Could you check a few things on this model? Use its own coordinates, in mm. Face numbers are marked on the shaded views. Give positions to 0.01 mm unless a question says otherwise; leave off trailing zeros. Write each loop counter-clockwise with the first axis right and the second up, starting at its lowest first coordinate (ties: lowest second). Pieces come first, ordered by that corner, then holes. Notation, with made-up numbers: M -29.5,-19.75 L 25.5,-19.75 A32 cw 25.5,17.25 Z; hole C 78,-19 d3. An arc over 180 degrees is marked long. Answer as CSV lines item,"result". Start each with the question number.
from build123d import *

# Parameters (mm, degrees)
SKETCH1_W         = 30
SKETCH1_H         = 30
EXTRUSION1_DEPTH  = 3.5
SKETCH2_W         = 80
SKETCH2_H         = 80
EXTRUSION2_DEPTH  = 8
EXTRUSION3_DEPTH  = 3.5
FILLET1_R         = 0.5
HOLE2_D           = 4.305
HOLE2_DEPTH       = 8
HOLE2_CBORE_D     = 7.145
HOLE2_CBORE_DEPTH = 4
HOLE2_TIP         = 1.293352482
EXTRUSION4_START  = 0.5
SKETCH6_R         = 3.5
SKETCH6_R_2       = 2.1525
EXTRUSION4_DEPTH  = 0.5


with BuildPart() as part:
    # Sketch1 → Extrusion1 (new body)
    with BuildSketch(Plane.XY):
        Rectangle(SKETCH1_W, SKETCH1_H)
    extrude(amount=EXTRUSION1_DEPTH)

    # Sketch2 → Extrusion2 (add)
    with BuildSketch(Plane(origin=(0, 0, 0), x_dir=(-1, 0, 0), z_dir=(0, 0, -1))):
        Rectangle(SKETCH2_W, SKETCH2_H)
    extrude(amount=EXTRUSION2_DEPTH)

    # Sketch3 → Extrusion3 (cut)
    with BuildSketch(Plane.XY.offset(3.5)):
        with BuildLine():
            Line((-2.292893219, -15), (2.292893219, -15))
            Line((2.292893219, -15), (2.292893219, -13.707106781))
            ThreePointArc((2.292893219, -13.707106781), (2, -13), (1.292893219, -12.707106781))
            Line((1.292893219, -12.707106781), (-1.292893219, -12.707106781))
            ThreePointArc((-1.292893219, -12.707106781), (-2, -13), (-2.292893219, -13.707106781))
            Line((-2.292893219, -13.707106781), (-2.292893219, -15))
        make_face()
    extrude(amount=-EXTRUSION3_DEPTH, mode=Mode.SUBTRACT)

    # Fillet1
    fillet1_edges = [part.edges().sort_by_distance(p)[0] for p in [
        (2.292893219, -15, 1.75),
        (-2.292893219, -15, 1.75),
        (-15, 15, 1.75),
        (15, 15, 1.75),
        (15, -15, 1.75),
        (-15, -15, 1.75),
    ]]
    fillet(fillet1_edges, radius=FILLET1_R)

    # Hole2
    with Locations(Plane(origin=(0, 0, -8), x_dir=(-1, 0, 0), z_dir=(0, 0, -1))):
        with Locations((24.525, -25.25), (24.525, 25.25), (-24.525, 25.25), (-24.525, -25.25)):
            CounterBoreHole(HOLE2_D / 2, HOLE2_CBORE_D / 2, HOLE2_CBORE_DEPTH, depth=HOLE2_DEPTH)
            with Locations((0, 0, -(HOLE2_DEPTH + HOLE2_TIP / 2))):  # 118° drill point
                Cone(0, HOLE2_D / 2, HOLE2_TIP, mode=Mode.SUBTRACT)

    # Sketch6 → Extrusion4 (add)
    # profile 1 of 4: a face of its own
    with BuildSketch(Plane.XY.offset(EXTRUSION4_START)):
        with Locations(Location((-24.525, 25.25, 0), (0, 0, 180))):
            Circle(SKETCH6_R)
        with Locations(Location((-24.525, 25.25, 0), (0, 0, 180))):
            Circle(SKETCH6_R_2, mode=Mode.SUBTRACT)
    # profile 2 of 4: a face of its own
    with BuildSketch(Plane.XY.offset(EXTRUSION4_START)):
        with Locations(Location((24.525, 25.25, 0), (0, 0, 180))):
            Circle(SKETCH6_R)
        with Locations(Location((24.525, 25.25, 0), (0, 0, 180))):
            Circle(SKETCH6_R_2, mode=Mode.SUBTRACT)
    # profile 3 of 4: a face of its own
    with BuildSketch(Plane.XY.offset(EXTRUSION4_START)):
        with Locations(Location((-24.525, -25.25, 0), (0, 0, 180))):
            Circle(SKETCH6_R)
        with Locations(Location((-24.525, -25.25, 0), (0, 0, 180))):
            Circle(SKETCH6_R_2, mode=Mode.SUBTRACT)
    # profile 4 of 4: a face of its own
    with BuildSketch(Plane.XY.offset(EXTRUSION4_START)):
        with Locations(Location((24.525, -25.25, 0), (0, 0, 180))):
            Circle(SKETCH6_R)
        with Locations(Location((24.525, -25.25, 0), (0, 0, 180))):
            Circle(SKETCH6_R_2, mode=Mode.SUBTRACT)
    extrude(amount=-EXTRUSION4_DEPTH)


solid = part.part
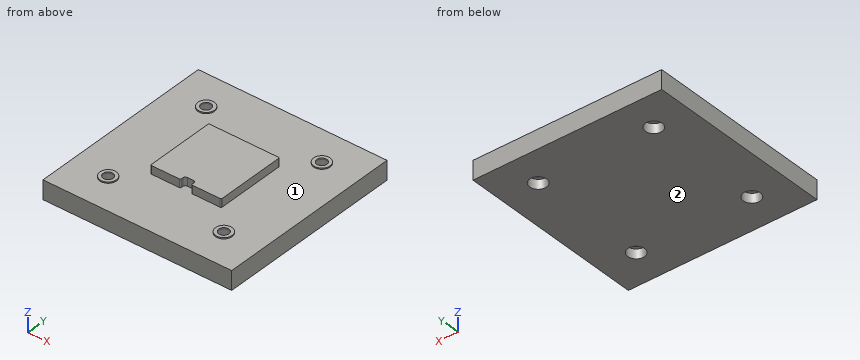
1. Imagine slicing it at A-A, the plane y = 25.25. Please give me the cut outline in (x, z) (1 decimal).
2. Please list where these lines run through material, in increasing order: line 1 (X direction, y = 25.5, z = -0.25); line 2 (X direction, y = -14.5, z = 3.25); line 3 (Y direction, x = -27, z = -5.5).
3. Will these pins go through, and if not, where does the flat tip stop? P1, Ø2.5, axis at x = 24.525, y = 25.25, coming from the -Z side; P2, Ø7, axis at x = 24.525, y = -25.25, coming from the -Z side; P3, Ø1.8, axis at x = 8.5, z = 1.5, coming from the -Y side; P4, Ø3, axis at x = 0.5, z = 2.5, coming from the -Y side.
4. Thinking about a two-plate mould opening in X: for the marked faces 1 and 2, which applies, pulls with the +X half, pulls with the -X half, needs draft (parallel to the pull), parting line crosses it, or undercut?
5. Imagine slicing it at B-B, the plane x = 16.5. Please give me the cut outline in (y, z).
Solutions:
1,outline,"M -40,-8 L -28.1,-8 L -28.1,-4 L -26.7,-4 L -26.7,0.5 L -28,0.5 L -28,0 L -40,0 Z; M -22.4,-4 L -21,-4 L -21,-8 L 21,-8 L 21,-4 L 22.4,-4 L 22.4,0.5 L 21,0.5 L 21,0 L -21,0 L -21,0.5 L -22.4,0.5 Z; M 26.7,-4 L 28.1,-4 L 28.1,-8 L 40,-8 L 40,0 L 28,0 L 28,0.5 L 26.7,0.5 Z"
2,line 1,"-40 to -26.66, -22.39 to 22.39, 26.66 to 40"
2,line 2,"-15 to -2.29, 2.29 to 15"
2,line 3,"-40 to -27.83, -22.67 to 22.67, 27.83 to 40"
3,P1,"through"
3,P2,"z = -4"
3,P3,"y = -15"
3,P4,"y = -13"
4,face 1,"undercut"
4,face 2,"needs draft"
5,outline,"M -40,-8 L 40,-8 L 40,0 L -40,0 Z"
